Source: CAD feature listing. Evaluate the final solid. Frame: model axes, mm. A direction names the side the tool comes from. Round coordinates to 2 decimals unless told otherwise and drop trailing zeros. Order: outer loops, then holes, each group sorted by start corner. A loop starts at its lowest first (then second) coordinate and runs counter-clockwise, first axis right, second up. Notation, with made-up numbers: (7, 69.5) - (32, 69.5) arc R25 cw to (32, 90.5) - close; hole circle Ø1 at (-20, 5.25). An arc over 180 degrees is marked (long way). Use one line per item in the form item = value. Start each with the question number.
Q1. Cut plane C-C, the plane y = 16.5. Return the cut outline in (x, z).
Q2. Pin query (flat end, axial travel): pin 1 Ø1.5 at (x, y) = (0, -10.38) entering from -Z; pin 2 Ø0.6 at (y, z) = (18.5, 1) entering from +X. Return the tip coordinate at first contact, or that it passes through.
Q3. Draft query along X for faces 1 (the cylindrical face through (12.437, -0.643, 0.986)), 2 (the cylindrical face through (4.641, 22.636, 0.986)), 3 (the flat face through (-5, -4, 2)). Return one class per face: released by +X, released by -X, zero draft, split by the parting line, or undercut.
Q4. Ray query, line 1 (Y direction, x = 0, z = 0.4); line 2 (X direction, y = -18.5, z = 1.6); line 3 (X direction, y = -10, z = 0.2). Return the intervals inside material, ascending. Write a range as [from, to].
Q5. Cut plane A-A, the plane x = 0. Return the cut outline in (y, z), and give its area (3 significant figures).
Q6. Set-up query: faces 4 (the flat face through (5.805, -17.07, 0.986)), 5 (the flat face through (-18.508, 0.686, 0.986)), 6 (the flat face through (-18.2, -3.304, 0.986)), 7 (the flat face through (9.311, 16.616, 0.986)). Return all of +Z, -Z, +X, -X, +Y, -Y with unobstructed straight access to the full face (end or side cutting, diameter ignored); none if empty.
Q7. Cut plane D-D, the plane z = 0.85. Give the number of separate pieces and of enclosed holes in the cut face, and give its area (3 significant figures).
Q8. Cut plane B-B, the plane y = -6. Return the cut outline in (x, z), and give its area (3 significant figures).
from build123d import *

# Parameters (mm, degrees)
SKETCH1_R                     = 1
SKETCH1_R_2                   = 6
BOSS_EXTRUDE1_DEPTH           = 2
CSK_FOR_M3_SFHCS1_D           = 2.5
CSK_FOR_M3_SFHCS1_DEPTH       = 9.5
CSK_FOR_M3_SFHCS1_CSINK_D     = 4
CSK_FOR_M3_SFHCS1_CSINK_ANGLE = 90
CSK_FOR_M3_SFHCS1_TIP         = 0.751075774


with BuildPart() as part:
    # Sketch1 → Boss-Extrude1 (new body)
    with BuildSketch(Plane(origin=(0, 0, 0), x_dir=(-1, 0, 0), z_dir=(0, 0, -1))):
        with BuildLine():
            Line((-15.316309042, 17.102154929), (-9.437338757, 11.808706309))
            ThreePointArc((-9.437338757, 11.808706309), (-9.289310319, 8.984155445), (-12.113861182, 8.836127007))
            Line((-12.113861182, 8.836127007), (-17.992831467, 14.129575627))
            ThreePointArc((-17.992831467, 14.129575627), (-19.485571585, 11.870022867), (-20.696031618, 9.447495623))
            Line((-20.696031618, 9.447495623), (-13.172285497, 7.002882316))
            ThreePointArc((-13.172285497, 7.002882316), (-11.888206454, 4.482735294), (-14.408353475, 3.198656251))
            Line((-14.408353475, 3.198656251), (-21.932099596, 5.643269556))
            ThreePointArc((-21.932099596, 5.643269556), (-22.376742646, 2.971913289), (-22.497222312, 0.266486078))
            Line((-22.497222312, 0.266486078), (-14.62962441, 1.093403939))
            ThreePointArc((-14.62962441, 1.093403939), (-12.431523692, -0.686582926), (-14.211510557, -2.884683643))
            Line((-14.211510557, -2.884683643), (-22.079108459, -3.711601503))
            ThreePointArc((-22.079108459, -3.711601503), (-21.398771617, -6.332859507), (-20.408438887, -8.853393742))
            Line((-20.408438887, -8.853393742), (-13.557368355, -4.897926326))
            ThreePointArc((-13.557368355, -4.897926326), (-10.825317547, -5.629977134), (-11.557368355, -8.362027942))
            Line((-11.557368355, -8.362027942), (-18.408438886, -12.317495358))
            ThreePointArc((-18.408438886, -12.317495358), (-16.720758571, -14.435415779), (-14.790850969, -16.335233771))
            Line((-14.790850969, -16.335233771), (-10.140920148, -9.935153049))
            ThreePointArc((-10.140920148, -9.935153049), (-7.347315654, -9.492689564), (-6.90485217, -12.286294058))
            Line((-6.90485217, -12.286294058), (-11.554782995, -18.686374777))
            ThreePointArc((-11.554782995, -18.686374777), (-9.151574469, -19.934749931), (-6.615790555, -20.885355888))
            Line((-6.615790555, -20.885355888), (-4.971014718, -13.147293963))
            ThreePointArc((-4.971014718, -13.147293963), (-2.598896135, -11.606822144), (-1.058424316, -13.978940727))
            Line((-1.058424316, -13.978940727), (-2.703200152, -21.717002651))
            ThreePointArc((-2.703200152, -21.717002651), (-3e-09, -21.879977134), (2.703200146, -21.717002651))
            Line((2.703200146, -21.717002651), (1.058424314, -13.978940725))
            ThreePointArc((1.058424314, -13.978940725), (2.598896135, -11.606822143), (4.971014718, -13.147293963))
            Line((4.971014718, -13.147293963), (6.615790554, -20.885355888))
            ThreePointArc((6.615790554, -20.885355888), (9.151574469, -19.934749931), (11.554782995, -18.686374777))
            Line((11.554782995, -18.686374777), (6.904852169, -12.286294058))
            ThreePointArc((6.904852169, -12.286294058), (7.347315653, -9.492689564), (10.140920146, -9.935153048))
            Line((10.140920146, -9.935153048), (14.790850972, -16.335233768))
            ThreePointArc((14.790850972, -16.335233768), (16.720758571, -14.435415779), (18.408438883, -12.317495361))
            Line((18.408438883, -12.317495361), (11.557368352, -8.362027946))
            ThreePointArc((11.557368352, -8.362027946), (10.825317543, -5.629977135), (13.557368354, -4.897926327))
            Line((13.557368354, -4.897926327), (20.408438886, -8.853393742))
            ThreePointArc((20.408438886, -8.853393742), (21.398771616, -6.332859507), (22.079108458, -3.711601502))
            Line((22.079108458, -3.711601502), (14.211510556, -2.884683643))
            ThreePointArc((14.211510556, -2.884683643), (12.431523691, -0.686582926), (14.629624409, 1.093403939))
            Line((14.629624409, 1.093403939), (22.497222311, 0.266486078))
            ThreePointArc((22.497222311, 0.266486078), (22.376742645, 2.971913287), (21.932099596, 5.643269552))
            Line((21.932099596, 5.643269552), (14.408353473, 3.19865625))
            ThreePointArc((14.408353473, 3.19865625), (11.888206452, 4.482735295), (13.172285497, 7.002882316))
            Line((13.172285497, 7.002882316), (20.696031618, 9.447495621))
            ThreePointArc((20.696031618, 9.447495621), (19.485571584, 11.870022866), (17.992831465, 14.129575628))
            Line((17.992831465, 14.129575628), (12.113861182, 8.836127007))
            ThreePointArc((12.113861182, 8.836127007), (9.289310318, 8.984155445), (9.437338756, 11.808706308))
            Line((9.437338756, 11.808706308), (15.316309041, 17.102154929))
            ThreePointArc((15.316309041, 17.102154929), (13.225168178, 18.822905238), (10.94243932, 20.279957294))
            Line((10.94243932, 20.279957294), (7.724772239, 13.052958714))
            ThreePointArc((7.724772239, 13.052958714), (5.084208037, 12.039341086), (4.070590408, 14.679905287))
            Line((4.070590408, 14.679905287), (7.288257486, 21.906903868))
            ThreePointArc((7.288257486, 21.906903868), (4.67801304, 22.628343883), (1.999999993, 23.030957697))
            Line((1.999999993, 23.030957697), (1.999999993, 15.120022866))
            ThreePointArc((1.999999993, 15.120022866), (-1e-09, 13.120022872), (-1.999999995, 15.120022866))
            Line((-1.999999995, 15.120022866), (-1.999999995, 23.030957697))
            ThreePointArc((-1.999999995, 23.030957697), (-4.67801304, 22.628343883), (-7.288257483, 21.906903869))
            Line((-7.288257483, 21.906903869), (-4.070590409, 14.679905287))
            ThreePointArc((-4.070590409, 14.679905287), (-5.084208039, 12.039341085), (-7.72477224, 13.052958715))
            Line((-7.72477224, 13.052958715), (-10.942439317, 20.279957296))
            ThreePointArc((-10.942439317, 20.279957296), (-13.225168177, 18.822905239), (-15.316309042, 17.102154929))
        make_face()
        with Locations(Location((9.526279442, 6.120022866, 0), (0, 0, 180))):
            Circle(SKETCH1_R, mode=Mode.SUBTRACT)
        with Locations(Location((-9.526279442, 6.120022866, 0), (0, 0, 180))):
            Circle(SKETCH1_R, mode=Mode.SUBTRACT)
        with Locations(Location((0, -10.379977134, 0), (0, 0, 180))):
            Circle(SKETCH1_R, mode=Mode.SUBTRACT)
        with Locations(Location((0, 0.620022866, 0), (0, 0, 180))):
            Circle(SKETCH1_R_2, mode=Mode.SUBTRACT)
    extrude(amount=-BOSS_EXTRUDE1_DEPTH)

    # CSK for M3 SFHCS1
    with Locations(Plane(origin=(-9.526279442, 6.120022866, 2), x_dir=(1, 0, 0), z_dir=(0, 0, 1))):
        with Locations((0, 0), (19.052558884, 0), (9.526279442, -16.5)):
            CounterSinkHole(CSK_FOR_M3_SFHCS1_D / 2, CSK_FOR_M3_SFHCS1_CSINK_D / 2, depth=CSK_FOR_M3_SFHCS1_DEPTH, counter_sink_angle=CSK_FOR_M3_SFHCS1_CSINK_ANGLE)
            with Locations((0, 0, -(CSK_FOR_M3_SFHCS1_DEPTH + CSK_FOR_M3_SFHCS1_TIP / 2))):  # 118° drill point
                Cone(0, CSK_FOR_M3_SFHCS1_D / 2, CSK_FOR_M3_SFHCS1_TIP, mode=Mode.SUBTRACT)


solid = part.part
Completed:
q1.outline = (-14.65, 0) - (-9.26, 0) - (-9.26, 2) - (-14.65, 2) - close; (-4.88, 0) - (-2, 0) - (-2, 2) - (-4.88, 2) - close; (2, 0) - (4.88, 0) - (4.88, 2) - (2, 2) - close; (9.26, 0) - (14.65, 0) - (14.65, 2) - (9.26, 2) - close
q2.pin_1 = through
q2.pin_2 = 14.04
q3.face_1 = undercut
q3.face_2 = released by +X
q3.face_3 = zero draft
q4.line_1 = [-21.88, -11.63], [-9.13, -5.38], [6.62, 13.12]
q4.line_2 = [-11.42, -6.11], [-2.02, 2.02], [6.11, 11.42]
q4.line_3 = [-14.39, -10.19], [-6.86, -1.19], [1.19, 6.86], [10.19, 14.39]
q5.outline = (-21.88, 0) - (-11.63, 0) - (-11.63, 1.25) - (-12.38, 2) - (-21.88, 2) - close; (-9.13, 0) - (-5.38, 0) - (-5.38, 2) - (-8.38, 2) - (-9.13, 1.25) - close; (6.62, 0) - (13.12, 0) - (13.12, 2) - (6.62, 2) - close
q5.area = 40.4 mm2
q6.face_4 = +Z, -Z, -Y
q6.face_5 = +Z, -Z
q6.face_6 = +Z, -Z, -X
q6.face_7 = +Z, -Z, +Y
q7.separate_pieces = 1
q7.enclosed_holes = 4
q7.area = 890 mm2
q8.outline = (-21.5, 0) - (-15.47, 0) - (-15.47, 2) - (-21.5, 2) - close; (-10.66, 0) - (10.66, 0) - (10.66, 2) - (-10.66, 2) - close; (15.47, 0) - (21.5, 0) - (21.5, 2) - (15.47, 2) - close
q8.area = 66.8 mm2
